The model under review builds one solid part; all positions refer to its coordinate system, in mm. Give positions to 0.01 mm unless a question says otherwise; leave off trailing zeros. Loops run counter-clockwise (first coordinate to the right, second up) from the corner with the lowest first, then second, coordinate; pieces in that order, holes last. Notation, with made-up numbers: M 13.5,56 L 25.5,56 A21 ccw 25.5,72 Z; hole C 10,44.25 d7. An arc over 180 degrees is marked long. Put each result on its own line as item: value. Start each with the question number.
```python
from build123d import *

# Parameters (mm, degrees)
SKETCH2_W           = 100
SKETCH2_H           = 100
BOSS_EXTRUDE1_DEPTH = 165
SKETCH3_W           = 70.5
SKETCH3_H           = 70.499969084
CUT_EXTRUDE1_DEPTH  = 164
CUT_EXTRUDE1_DRAFT  = -2


with BuildPart() as part:
    # Sketch2 → Boss-Extrude1 (new body)
    with BuildSketch(Plane.XZ.offset(2.5)):
        Rectangle(SKETCH2_W, SKETCH2_H)
    extrude(amount=BOSS_EXTRUDE1_DEPTH)


with BuildPart() as cut_extrude1_tool:
    # Sketch3 → Cut-Extrude1 (with draft: the straight prism first)
    with BuildSketch(Plane(origin=(0, -2.5, 0), x_dir=(1, 0, 0), z_dir=(0, 1, 0))):
        Rectangle(SKETCH3_W, SKETCH3_H)
    extrude(amount=-CUT_EXTRUDE1_DEPTH)
    # Cut-Extrude1: the draft: its side faces are tilted about the plane it starts from
    cut_extrude1_sides = [cut_extrude1_tool.faces().sort_by_distance(p)[0] for p in [
        (0, -84.5, 35.249984542),
        (35.25, -84.5, 0),
        (0, -84.5, -35.249984542),
        (-35.25, -84.5, 0),
    ]]
    draft(cut_extrude1_sides, Plane(origin=(0, -2.5, 0), x_dir=(1, 0, 0), z_dir=(0, 1, 0)), CUT_EXTRUDE1_DRAFT)


with BuildPart() as part_1:
    add(part.part)

    # Cut-Extrude1: cut by cut_extrude1_tool
    add(cut_extrude1_tool.part, mode=Mode.SUBTRACT)


solid = part_1.part
```
Item 1: Consider section A-A, the plane y = -118.5. Write out the cut boundary in (x, z).
Item 2: Consider section B-B, the plane x = -8.5. Write out the cut boundary in (y, z), plus the area to 3 significant figures.
Item 3: Draft analysis for pull direction Z (two halves, no side actions). For faces 1 (the flat face through (-1, -84, 50)), 2 (the flat face through (-1, -167.5, 1)), 3 (the flat face through (0, -166.5, 0)), state which applies: +Z half, -Z half, draft (parallel to the pull), parting line (faces both ways), or undercut.
Item 4: Consider section C-C, the plane z = 24. Write out the cut boundary in (x, y), plus the area to 3 significant figures.
Item 5: Consider section D-D, the plane y = -152. Write out the cut boundary in (x, z), plus the area to 3 significant figures.
Item 6: To check wall thickness, follow L1, parallel to Y at x = 8.5, z = -27.5; L2, parallel to X at y = -59, z = 11; L3, parallel to X at y = -43, z = 15. State the ranges of each line that lie inside material, in increasing order. Write a range as [from, to].
Report:
1. outline: M -50,-50 L 50,-50 L 50,50 L -50,50 Z; hole M -31.2,-31.2 L 31.2,-31.2 L 31.2,31.2 L -31.2,31.2 Z
2. outline: M -167.5,-50 L -2.5,-50 L -2.5,-35.25 L -166.5,-29.52 L -166.5,29.52 L -2.5,35.25 L -2.5,50 L -167.5,50 Z
2. area: 5,880 mm²
3. face 1: +Z half
3. face 2: draft
3. face 3: undercut
4. outline: M -50,-167.5 L 50,-167.5 L 50,-2.5 L 35.25,-2.5 L 29.52,-166.5 L -29.52,-166.5 L -35.25,-2.5 L -50,-2.5 Z
4. area: 5,880 mm²
5. outline: M -50,-50 L 50,-50 L 50,50 L -50,50 Z; hole M -30.03,-30.03 L 30.03,-30.03 L 30.03,30.03 L -30.03,30.03 Z
5. area: 6,390 mm²
6. L1: [-167.5, -166.5]
6. L2: [-50, -33.28], [33.28, 50]
6. L3: [-50, -33.84], [33.84, 50]
